The model under review builds one solid part; all positions refer to its coordinate system, in mm. Face numbers are marked on the shaded views. A direction names the side the tool comes from. Give positions to 0.01 mm unless a question says otherwise; leave off trailing zeros. Loops run counter-clockwise (first coordinate to the right, second up) from the corner with the lowest first, then second, coordinate; pieces in that order, holes last. Notation, with made-up numbers: (7, 18.25) - (18, 18.25) arc R13 cw to (18, 37.25) - close; hole circle Ø6 at (18, 66.5). An arc over 180 degrees is marked (long way). Answer as a JSON object with one key per item and string values.
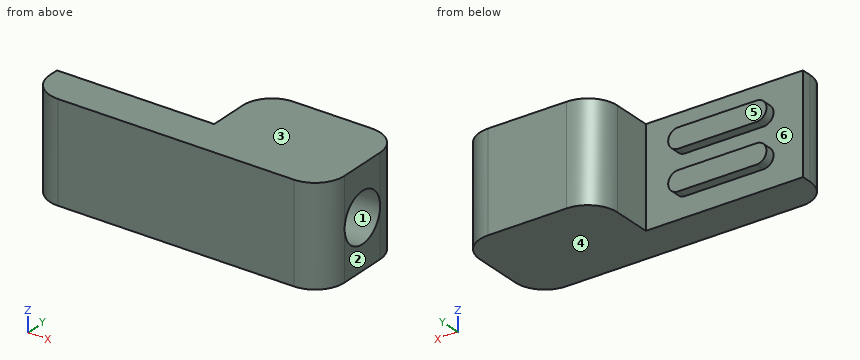
from build123d import *

# Parameters (mm, degrees)
EXTRUDE_1_DEPTH        = 2.5
FILLET_1_R             = 1.5
HOLE_WIZARD_M3_1_D     = 2.5
HOLE_WIZARD_M3_1_DEPTH = 5
HOLE_WIZARD_M3_1_TIP   = 0.751075774
EXTRUDE_2_DEPTH        = 0.5


with BuildPart() as part:
    # 스케치1 → 보스-돌출1 (new body, symmetric)
    with BuildSketch(Plane.XY):
        Polygon((0, 0), (-15, 0), (-15, 2), (-7, 2), (-7, 5.5), (0, 5.5), align=None)
    extrude(amount=EXTRUDE_1_DEPTH, both=True)

    # 필렛1
    fillet_1_edges = [part.edges().sort_by_distance(p)[0] for p in [
        (0, 0, 0),
        (-15, 0, 0),
        (-7, 5.5, 0),
        (0, 5.5, 0),
    ]]
    fillet(fillet_1_edges, radius=FILLET_1_R)

    # M3 나사 구멍1
    with Locations(Plane(origin=(0, 0, 0), x_dir=(0, 0, -1), z_dir=(1, 0, 0))):
        with Locations((0, 2.75)):
            Hole(HOLE_WIZARD_M3_1_D / 2, depth=HOLE_WIZARD_M3_1_DEPTH)
            with Locations((0, 0, -(HOLE_WIZARD_M3_1_DEPTH + HOLE_WIZARD_M3_1_TIP / 2))):  # 118° drill point
                Cone(0, HOLE_WIZARD_M3_1_D / 2, HOLE_WIZARD_M3_1_TIP, mode=Mode.SUBTRACT)

    # 스케치4 → 보스-돌출2 (add)
    with BuildSketch(Plane(origin=(0, 2, 0), x_dir=(1, 0, 0), z_dir=(0, 1, 0))):
        with BuildLine():
            Line((-13, 1.5), (-9, 1.5))
            ThreePointArc((-9, 1.5), (-8.5, 1), (-9, 0.5))
            Line((-9, 0.5), (-13, 0.5))
            ThreePointArc((-13, 0.5), (-13.5, 1), (-13, 1.5))
        make_face()
        with BuildLine():
            Line((-13, -1.5), (-9, -1.5))
            ThreePointArc((-9, -1.5), (-8.5, -1), (-9, -0.5))
            Line((-9, -0.5), (-13, -0.5))
            ThreePointArc((-13, -0.5), (-13.5, -1), (-13, -1.5))
        make_face()
    extrude(amount=EXTRUDE_2_DEPTH)


solid = part.part
Q1. The part is to be moulded in two halves that separate along Z. For the marked faces 1, 2 and 3, say which applies: +Z half, -Z half, draft (parallel to the pull), parting line (faces both ways), or undercut.
Results:
{"face 1": "undercut", "face 2": "draft", "face 3": "+Z half"}
Q2. To check wall thickness, follow probe 1 along Y at (x, z) = (-3.3, 0); probe 2 along Z at (x, y) = (-3, 2.75); probe 3 along X at (y, z) = (2.85, 1.6). State the ranges of each line that lie inside material, in increasing order. Write a range as [from, to].
Results:
{"probe 1": "y = [0, 1.5], [4, 5.5]", "probe 2": "z = [-2.5, -1.25], [1.25, 2.5]", "probe 3": "x = [-7, 0]"}
Q3. Consider section A-A, the plane z = -1.85. State the section outline as (x, y) points, plus the area to 3 significant figures.
Results:
{"outline": "(-15, 1.5) arc R1.5 ccw to (-13.5, 0) - (-1.5, 0) arc R1.5 ccw to (0, 1.5) - (0, 4) arc R1.5 ccw to (-1.5, 5.5) - (-5.5, 5.5) arc R1.5 ccw to (-7, 4) - (-7, 2) - (-15, 2) - close", "area": "52.6 mm^2"}
Q4. Consider section B-B, the plane x = -5.25. State the section outline as (y, z) points, plus the area to 3 significant figures.
Results:
{"outline": "(0, -2.5) - (5.5, -2.5) - (5.5, 2.5) - (0, 2.5) - close; hole circle Ø1.67 at (2.75, 0)", "area": "25.3 mm^2"}
Q5. Clearance check with flat-ended pins moving along their axes: pin 1 Ø1.1 at (x, z) = (-10.5, 1) entering from +Y; pin 2 Ø0.6 at (x, y) = (-11.5, 2.5) entering from +Z. State where each tip first meets the part, or that it passes through.
Results:
{"pin 1": "stops at y = 2.5", "pin 2": "stops at z = 1.5"}
Q6. For the marked faces 4, 5 and 6, list the 3-axis set-ups (+Z, -Z, +X, -X, +Y, -Y) from which the entire face can be reached by the end or side of a thin tool; tool diameter is ignored.
Results:
{"face 4": "-Z, +X, -X, +Y, -Y", "face 5": "+Z, -Z, -X, +Y", "face 6": "+Y"}
Q7. Consider section C-C, the plane x = -7.75. State the section outline as (y, z) points, plus the area to 3 significant figures.
Results:
{"outline": "(0, -2.5) - (2, -2.5) - (2, 2.5) - (0, 2.5) - close", "area": "10.0 mm^2"}
Q8. Consider section D-D, the plane y = 4.4. State the section outline as (x, z) points.
Results:
{"outline": "(-6.95, -2.5) - (-0.05, -2.5) - (-0.05, 2.5) - (-6.95, 2.5) - close"}
